Build history of the part. All positions in model axes, mm. A direction names the side the tool comes from. Give positions to 0.01 mm unless a question says otherwise; leave off trailing zeros. Loops run counter-clockwise (first coordinate to the right, second up) from the corner with the lowest first, then second, coordinate; pieces in that order, holes last. Notation, with made-up numbers: (15, 12.25) -> (37, 12.25) arc R7 cw to (37, 24.25) -> close; hole circle Ø9 at (62, -26). An arc over 180 degrees is marked (long way). Answer as a JSON object with one key per item and string values. Group by question number.
from build123d import *

# Parameters (mm, degrees)
BOSS_EXTRUDE1_DEPTH      = 25.4
BOSS_EXTRUDE1_DEPTH_BACK = 34.925
CUT_EXTRUDE4_DEPTH       = 63.941922635
CUT_EXTRUDE5_DEPTH       = 46.01339384
SKETCH14_R               = 3.2893
CUT_EXTRUDE6_DEPTH       = 46.01339384
CUT_EXTRUDE7_DEPTH       = 76.2
CUT_EXTRUDE7_DEPTH_BACK  = 12.7
SKETCH15_R               = 12.7
CUT_EXTRUDE8_DEPTH       = 10.668
CUT_EXTRUDE8_DEPTH_BACK  = 25.4
SKETCH16_R               = 12.7
CUT_EXTRUDE9_DEPTH       = 13.462
CUT_EXTRUDE9_DEPTH_BACK  = 25.4
SKETCH17_R               = 12.7
CUT_EXTRUDE10_DEPTH      = 11.43
CUT_EXTRUDE10_DEPTH_BACK = 25.4
SKETCH18_R               = 12.7
CUT_EXTRUDE11_DEPTH      = 10.668
CUT_EXTRUDE11_DEPTH_BACK = 25.4
SKETCH19_R               = 12.7
SKETCH20_W               = 46.918980947
SKETCH20_H               = 36.132247669
CUT_EXTRUDE12_DEPTH      = 51.98499249


with BuildPart() as part:
    # Sketch1 → Boss-Extrude1 (new, two sides: drawn at the far end of the back side and taken through both)
    with BuildSketch(Plane(origin=(0, 0, 0), x_dir=(0, 0, -1), z_dir=(1, 0, 0)).offset(-BOSS_EXTRUDE1_DEPTH_BACK)):
        with BuildLine():
            Line((-10.16, 12.7), (10.16, 12.7))
            ThreePointArc((10.16, 12.7), (11.956051224, 11.956051224), (12.7, 10.16))
            Line((12.7, 10.16), (12.7, -10.16))
            ThreePointArc((12.7, -10.16), (11.956051224, -11.956051224), (10.16, -12.7))
            Line((10.16, -12.7), (-10.16, -12.7))
            ThreePointArc((-10.16, -12.7), (-11.956051224, -11.956051224), (-12.7, -10.16))
            Line((-12.7, -10.16), (-12.7, 10.16))
            ThreePointArc((-12.7, 10.16), (-11.956051224, 11.956051224), (-10.16, 12.7))
        make_face()
    extrude(amount=BOSS_EXTRUDE1_DEPTH + BOSS_EXTRUDE1_DEPTH_BACK)

    # Sketch11 → Cut-Extrude4 (cut, through all)
    with BuildSketch(Plane(origin=(25.4, 0, 0), x_dir=(0, 0, -1), z_dir=(1, 0, 0))):
        with BuildLine():
            Line((-10.6045, 11.1125), (10.6045, 11.1125))
            ThreePointArc((10.6045, 11.1125), (10.963710245, 10.963710245), (11.1125, 10.6045))
            Line((11.1125, 10.6045), (11.1125, -10.6045))
            ThreePointArc((11.1125, -10.6045), (10.963710245, -10.963710245), (10.6045, -11.1125))
            Line((10.6045, -11.1125), (-10.6045, -11.1125))
            ThreePointArc((-10.6045, -11.1125), (-10.963710245, -10.963710245), (-11.1125, -10.6045))
            Line((-11.1125, -10.6045), (-11.1125, 10.6045))
            ThreePointArc((-11.1125, 10.6045), (-10.963710245, 10.963710245), (-10.6045, 11.1125))
        make_face()
    extrude(amount=-CUT_EXTRUDE4_DEPTH, mode=Mode.SUBTRACT)

    # Sketch12 → Cut-Extrude5 (cut, through all)
    with BuildSketch(Plane(origin=(0, 12.7, 0), x_dir=(1, 0, 0), z_dir=(0, 1, 0))):
        with BuildLine():
            Line((0, 12.7), (50.8, 12.7))
            Line((50.8, 12.7), (50.8, -12.7))
            Line((50.8, -12.7), (0, -12.7))
            Line((0, -12.7), (19.444424463, -7.686083637))
            ThreePointArc((19.444424463, -7.686083637), (25.4, 0), (19.444424463, 7.686083637))
            Line((19.444424463, 7.686083637), (0, 12.7))
        make_face()
    extrude(amount=-CUT_EXTRUDE5_DEPTH, mode=Mode.SUBTRACT)

    # Sketch14 → Cut-Extrude6 (cut, through all)
    with BuildSketch(Plane(origin=(0, 12.7, 0), x_dir=(1, 0, 0), z_dir=(0, 1, 0))):
        with Locations(Location((17.4625, 0, 0), (0, 0, 270))):
            Circle(SKETCH14_R)
    extrude(amount=-CUT_EXTRUDE6_DEPTH, mode=Mode.SUBTRACT)

    # Sketch15 → Cut-Extrude7 (cut, two sides: drawn at the far end of the back side and taken through both)
    with BuildSketch(Plane(origin=(-25.365699209, 12.7, 0.175387953), x_dir=(-0.966128643141705, -0.2580531152287385, -0.0020086368292109116), z_dir=(0.258060932535648, -0.9660993767043435, -0.007519935525699624)).offset(-CUT_EXTRUDE7_DEPTH_BACK)):
        with Locations(Location((0, 0, 0), (0, 0, 319.301782521))):
            Circle(SKETCH15_R)
    extrude(amount=CUT_EXTRUDE7_DEPTH + CUT_EXTRUDE7_DEPTH_BACK, mode=Mode.SUBTRACT)

    # Sketch16 → Cut-Extrude8 (cut, two sides: drawn at the far end of the back side and taken through both)
    with BuildSketch(Plane(origin=(-21.145247559, 12.7, -1.764300444), x_dir=(-0.9824624854144782, 0.18269743061253008, -0.03727081432952601), z_dir=(-0.18646035705534364, -0.9626355681875568, 0.1963804931937318)).offset(-CUT_EXTRUDE8_DEPTH_BACK)):
        Circle(SKETCH16_R)
    extrude(amount=CUT_EXTRUDE8_DEPTH + CUT_EXTRUDE8_DEPTH_BACK, mode=Mode.SUBTRACT)

    # Sketch17 → Cut-Extrude9 (cut, two sides: drawn at the far end of the back side and taken through both)
    with BuildSketch(Plane(origin=(-34.925, 0.334385976, 0.104098467), x_dir=(0, 0, -1), z_dir=(0.9661266940476223, 0.2580682294444866, 0)).offset(-CUT_EXTRUDE9_DEPTH_BACK)):
        Circle(SKETCH17_R)
    extrude(amount=CUT_EXTRUDE9_DEPTH + CUT_EXTRUDE9_DEPTH_BACK, mode=Mode.SUBTRACT)


with BuildPart() as body_2:
    # of the pieces the cut leaves, the one that is kept (cut_extrude9_keep)
    add(part.part.solids().sort_by_distance((-34.925, -12.7, 10.16))[0])

    # Sketch18 → Cut-Extrude10 (cut, two sides: drawn at the far end of the back side and taken through both)
    with BuildSketch(Plane(origin=(-21.542643879, 3.81098788, 12.7), x_dir=(-0.9940833845942291, 0.0023249747136513278, 0.10859474649476883), z_dir=(-0.1086196320822448, -0.021278093914850475, -0.9938556324968274)).offset(-CUT_EXTRUDE10_DEPTH_BACK)):
        Circle(SKETCH18_R)
    extrude(amount=CUT_EXTRUDE10_DEPTH + CUT_EXTRUDE10_DEPTH_BACK, mode=Mode.SUBTRACT)

    # Sketch19 → Cut-Extrude11 (cut, two sides: drawn at the far end of the back side and taken through both)
    with BuildSketch(Plane(origin=(-19.809355594, -2.656223175, 12.7), x_dir=(-0.9763290145154151, -0.09548845507502762, 0.19407114768234568), z_dir=(-0.2162906734359075, 0.43103175814294675, -0.8760308031438403)).offset(-CUT_EXTRUDE11_DEPTH_BACK)):
        Circle(SKETCH19_R)
    extrude(amount=CUT_EXTRUDE11_DEPTH + CUT_EXTRUDE11_DEPTH_BACK, mode=Mode.SUBTRACT)

    # Sketch20 → Cut-Extrude12 (cut, through all)
    with BuildSketch(Plane(origin=(-20.509915766, -5.478533696, 0), x_dir=(0.2580609325356479, -0.9660993767043435, -0.007519935525699628), z_dir=(-0.9661266940476223, -0.25806822944448654, 0))):
        with Locations((-1.610495454, -1.756475899)):
            Rectangle(SKETCH20_W, SKETCH20_H)
    extrude(amount=CUT_EXTRUDE12_DEPTH, mode=Mode.SUBTRACT)


solid = body_2.part
(1) Pull direction Y, two halves, no side cores. Call faces 3 (the cylindrical face through (-3.17, -12.26, 11.59)), 4 (the flat face through (-9, 0, -12.7)), 5 (the cylindrical face through (-7.08, -5.19, 11.61)): pulls with the +Y half, pulls with the -Y half, needs draft (parallel to the pull), parting line crosses it, or undercut.
(2) Probe line 1 along Z through (x, y) = (-2.5, 7.75); line 2 along Z through (x, y) = (-9, -8.5). List the from-to ranges inside material, lowest first. Write a range as [from, to].
(3) Saw through at A-A on x = 12.5. List the corners of the cut face in (y, z).
(4) 3-axis set-ups, long thin cutter, end or side, ignore diameter. For faces 1 (the flat face through (-5, 0, -11.112)), 2 (the flat face through (7, -12.7, 0)): which of +Z, -Z, +X, -X, +Y, -Y reach the whole face in a straight line?
(5) Saw through at B-B on z = -0.5. Give the number of separate pieces and of enclosed holes in the cut face, plus the area to 3 significant figures.
(6) Pin check, flat tip, straight feed: pin 1 (1 mm diameter, centred on x = 8, y = 6, fed in from -Z). Stop position of the tip, or through.
Calculated:
{
 "1": {"face 3": "pulls with the -Y half", "face 4": "needs draft", "face 5": "undercut"},
 "2": {"line 1": "z = [-12.7, -11.11], [11.11, 12.7]", "line 2": "z = [-12.7, -11.11]"},
 "3": {"outline": "(-12.7, -9.48) -> (-11.11, -9.48) -> (-11.11, 9.48) -> (-12.7, 9.48) -> close; (11.11, -9.48) -> (12.7, -9.48) -> (12.7, 9.48) -> (11.11, 9.48) -> close"},
 "4": {"face 1": "+X, -X", "face 2": "+Z, -Z, +X, -X, -Y"},
 "5": {"separate pieces": "4", "enclosed holes": "0", "area": "82.4 mm^2"},
 "6": {"pin 1": "passes through"}
}
